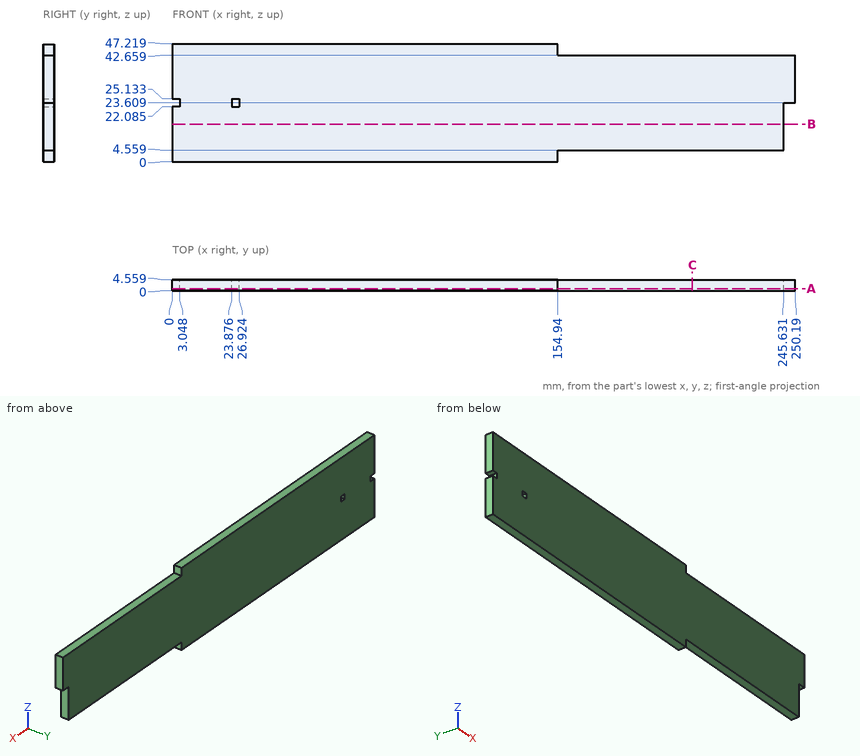
Source: three-view drawing plus pictorial views. Frame: mm from the lowest corner of the part. Coordinates: 2 decimals unless noted, no trailing zeros. Write each loop counter-clockwise with the first axis right and the second up, starting at its lowest first coordinate (ties: lowest second). Pieces come first, ordered by that corner, then holes. Notation, with made-up numbers: (73, 78.25) - (95, 78.25) arc R11 ccw to (95, 95.25) - close; hole circle Ø7 at (84.25, -27.75). An arc over 180 degrees is marked (long way). Return JSON: item names as keys, results as strings.
Item 1: Line query: L1, parallel to X at y = 0.65, z = 23; L2, parallel to Z at x = 229, y = 0.65; L3, parallel to X at y = 3, z = 4. Output: solid intervals per line, ascending.
Completed:
{"L1": "x = 3.05 to 23.88, 26.92 to 245.63", "L2": "z = 4.56 to 42.66", "L3": "x = 0 to 154.94"}
Item 2: Section query C-C (x = 209). Output: boundary loops of the cut face in (y, z).
Completed:
{"outline": "(0, 4.56) - (4.56, 4.56) - (4.56, 42.66) - (0, 42.66) - close"}
Item 3: Section query B-B (z = 15). Output: boundary loops of the cut face in (x, y), and give its area (3 significant figures).
Completed:
{"outline": "(0, 0) - (245.63, 0) - (245.63, 4.56) - (0, 4.56) - close", "area": "1,120 mm2"}
Item 4: Section query A-A (y = 0.9). Output: boundary loops of the cut face in (x, z) (1 decimal).
Completed:
{"outline": "(0, 0) - (154.9, 0) - (154.9, 4.6) - (245.6, 4.6) - (245.6, 23.6) - (250.2, 23.6) - (250.2, 42.7) - (154.9, 42.7) - (154.9, 47.2) - (0, 47.2) - (0, 25.1) - (3, 25.1) - (3, 22.1) - (0, 22.1) - close; hole (23.9, 22.1) - (26.9, 22.1) - (26.9, 25.1) - (23.9, 25.1) - close"}
Item 5: Pin query (flat end, axial travel): pin 1 Ø2.5 at (y, z) = (2.5, 2.5) entering from +X; pin 2 Ø2.5 at (x, y) = (220, 3.5) entering from +Z; pin 3 Ø1.5 at (y, z) = (3, 20) entering from +X. Return the tip coordinate at first contact, or that it passes through.
Completed:
{"pin 1": "stops at x = 154.94", "pin 2": "stops at z = 42.66", "pin 3": "stops at x = 245.63"}
